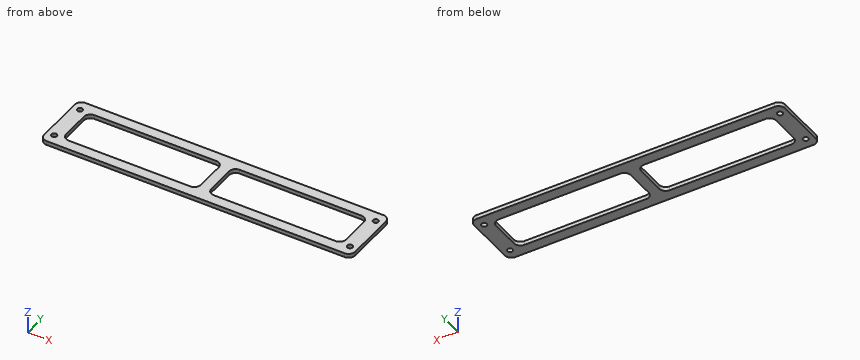
```python
from build123d import *

# Parameters (mm, degrees)
SKETCH1_W           = 238
SKETCH1_H           = 48
SKETCH1_R           = 2.05
SKETCH1_W_2         = 103.125
SKETCH1_H_2         = 32
BOSS_EXTRUDE1_DEPTH = 3.125
FILLET1_R           = 5


with BuildPart() as part:
    # Sketch1 → Boss-Extrude1 (new body)
    with BuildSketch(Plane.XY):
        Rectangle(SKETCH1_W, SKETCH1_H)
        with Locations((-113.175, 16)):
            Circle(SKETCH1_R, mode=Mode.SUBTRACT)
        with Locations((-113.175, -16)):
            Circle(SKETCH1_R, mode=Mode.SUBTRACT)
        with Locations((113.175, 16)):
            Circle(SKETCH1_R, mode=Mode.SUBTRACT)
        with Locations((113.175, -16)):
            Circle(SKETCH1_R, mode=Mode.SUBTRACT)
        with Locations((-55.5625, 0)):
            Rectangle(SKETCH1_W_2, SKETCH1_H_2, mode=Mode.SUBTRACT)
        with Locations((55.5625, 0)):
            Rectangle(SKETCH1_W_2, SKETCH1_H_2, mode=Mode.SUBTRACT)
    extrude(amount=BOSS_EXTRUDE1_DEPTH)

    # Fillet1
    fillet1_edges = [part.edges().sort_by_distance(p)[0] for p in [
        (-107.125, 16, 1.5625),
        (-107.125, -16, 1.5625),
        (-4, -16, 1.5625),
        (-4, 16, 1.5625),
        (107.125, -16, 1.5625),
        (107.125, 16, 1.5625),
        (4, 16, 1.5625),
        (4, -16, 1.5625),
        (-119, 24, 1.5625),
        (119, 24, 1.5625),
        (119, -24, 1.5625),
        (-119, -24, 1.5625),
    ]]
    fillet(fillet1_edges, radius=FILLET1_R)


solid = part.part
```
Part model, mm, in its own coordinate system. Coordinates: 2 decimals unless noted, no trailing zeros. Order: outer loops, then holes, each group sorted by start corner. A loop starts at its lowest first (then second) coordinate and runs counter-clockwise, first axis right, second up. Notation, with made-up numbers: (-2.5, 42.25) - (2.5, 42.25) arc R20 cw to (2.5, 68.25) - close; hole circle Ø7 at (77.25, -2.75). An arc over 180 degrees is marked (long way). Return JSON: item names as keys, results as strings. Group by question number.
Item 1: Cut at A-A (y = -5). List the corners of the cut face in (x, z) (3 decimals), plus the area to 3 significant figures.
Item 2: Drill centre lines: probe 1 along X at (y, z) = (-10, 1.7) (3 decimals); probe 2 along Y at (x, z) = (20, 2.65); probe 3 along X at (y, z) = (16.5, 1.6). Where is each one in solid material? Low to high. Write a range as from..to.
Item 3: Cut at B-B (x = -65.5). List the corners of the cut face in (y, z) (3 decimals).
Item 4: Cut at C-C (z = 2). List the corners of the cut face in (x, y) (3 decimals).
Item 5: Pin check, flat tip, straight feed: pin 1 (5 mm diameter, centred on x = -8.5, y = -5, fed in from -Z). Stop position of the tip, or through.
Check values:
{
 "1": {"outline": "(-119, 0) - (-107.125, 0) - (-107.125, 3.125) - (-119, 3.125) - close; (-4, 0) - (4, 0) - (4, 3.125) - (-4, 3.125) - close; (107.125, 0) - (119, 0) - (119, 3.125) - (107.125, 3.125) - close", "area": "99.2 mm2"},
 "2": {"probe 1": "x = -119..-107.125, -4..4, 107.125..119", "probe 2": "y = -24..-16, 16..24", "probe 3": "x = -119..-115.16, -111.19..111.19, 115.16..119"},
 "3": {"outline": "(-24, 0) - (-16, 0) - (-16, 3.125) - (-24, 3.125) - close; (16, 0) - (24, 0) - (24, 3.125) - (16, 3.125) - close"},
 "4": {"outline": "(-119, -19) arc R5 ccw to (-114, -24) - (114, -24) arc R5 ccw to (119, -19) - (119, 19) arc R5 ccw to (114, 24) - (-114, 24) arc R5 ccw to (-119, 19) - close; hole circle Ø4.1 at (-113.175, -16); hole circle Ø4.1 at (-113.175, 16); hole (-107.125, -11) arc R5 ccw to (-102.125, -16) - (-9, -16) arc R5 ccw to (-4, -11) - (-4, 11) arc R5 ccw to (-9, 16) - (-102.125, 16) arc R5 ccw to (-107.125, 11) - close; hole (4, -11) arc R5 ccw to (9, -16) - (102.125, -16) arc R5 ccw to (107.125, -11) - (107.125, 11) arc R5 ccw to (102.125, 16) - (9, 16) arc R5 ccw to (4, 11) - close; hole circle Ø4.1 at (113.175, -16); hole circle Ø4.1 at (113.175, 16)"},
 "5": {"pin 1": "passes through"}
}
